Part model, mm, in its own coordinate system. Coordinates: 2 decimals unless noted, no trailing zeros. Loops run counter-clockwise (first coordinate to the right, second up) from the corner with the lowest first, then second, coordinate; pieces in that order, holes last. Notation, with made-up numbers: (-7.5, -26) - (-1.5, -26) arc R29 cw to (-1.5, -2) - close; hole circle Ø2 at (-30.5, 41). An arc over 180 degrees is marked (long way). One line per question, with ' | ' between items. Start each with the question number.
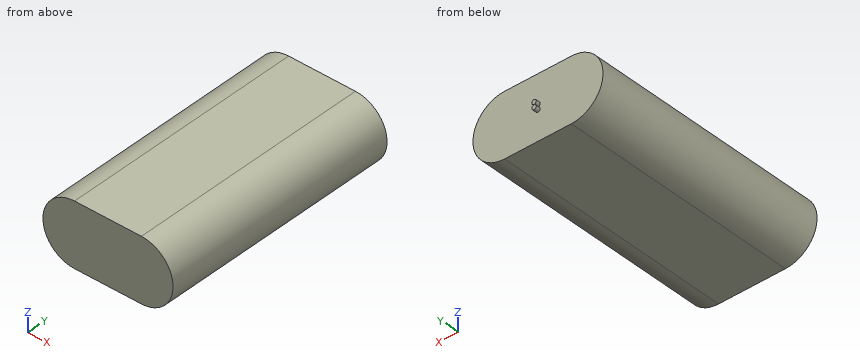
from build123d import *

# Parameters (mm, degrees)
SKETCH1_W           = 19
SKETCH1_H           = 18
BOSS_EXTRUDE1_DEPTH = 69
SKETCH2_R           = 0.635
BOSS_EXTRUDE2_DEPTH = 1.27
SKETCH3_R           = 0.635
BOSS_EXTRUDE4_DEPTH = 1.27


with BuildPart() as part:
    # Sketch1 → Boss-Extrude1 (new body)
    with BuildSketch(Plane(origin=(0, 0, 0), x_dir=(1, 0, 0), z_dir=(0, 1, 0))):
        with BuildLine():
            Line((0, 0), (0, 18))
            ThreePointArc((0, 18), (-9, 9), (0, 0))
        make_face()
        with Locations((9.5, 9)):
            Rectangle(SKETCH1_W, SKETCH1_H)
        with BuildLine():
            Line((19, 0), (19, 18))
            ThreePointArc((19, 18), (28, 9), (19, 0))
        make_face()
    extrude(amount=BOSS_EXTRUDE1_DEPTH)

    # Sketch2 → Boss-Extrude2 (add)
    with BuildSketch(Plane(origin=(0, 69, 0), x_dir=(1, 0, 0), z_dir=(0, 1, 0))):
        with Locations(Location((9.5, 9.635, 0), (0, 0, 270))):
            Circle(SKETCH2_R)
    extrude(amount=BOSS_EXTRUDE2_DEPTH)

    # Sketch3 → Boss-Extrude4 (add)
    with BuildSketch(Plane(origin=(0, 69, 0), x_dir=(1, 0, 0), z_dir=(0, 1, 0))):
        with Locations(Location((9.5, 8.238, 0), (0, 0, 270))):
            Circle(SKETCH3_R)
    extrude(amount=BOSS_EXTRUDE4_DEPTH)


solid = part.part
1) Wall check: line 1 along Y through (x, z) = (6, -12); line 2 along X through (y, z) = (62, -13.25); line 3 along X through (y, z) = (16, -17). Give the ranges that are in metal, low to high. Write a range as [from, to].
2) Band-saw the part on A-A on y = 51. List the corners of the cut face in (x, z), then the cut area to 3 significant figures.
3) Pin check, flat tips, straight feed: pin 1 Ø2 at (y, z) = (16.5, -7.5) entering from +X; pin 2 Ø3 at (y, z) = (31.5, -5) entering from -X; pin 3 Ø4 at (y, z) = (10, -13) entering from -X. Stop position of each tip, or through.
4) Band-saw the part on B-B on x = 6. List the corners of the cut face in (y, z), then the cut area to 3 significant figures.
Values found:
1) line 1: [0, 69] | line 2: [-7.93, 26.93] | line 3: [-4.12, 23.12]
2) outline: (0, -18) - (19, -18) arc R9 ccw to (19, 0) - (0, 0) arc R9 ccw to start | area: 596 mm²
3) pin 1: x = 27.99 | pin 2: x = -8.65 | pin 3: x = -8.77
4) outline: (0, -18) - (69, -18) - (69, 0) - (0, 0) - close | area: 1,240 mm²
